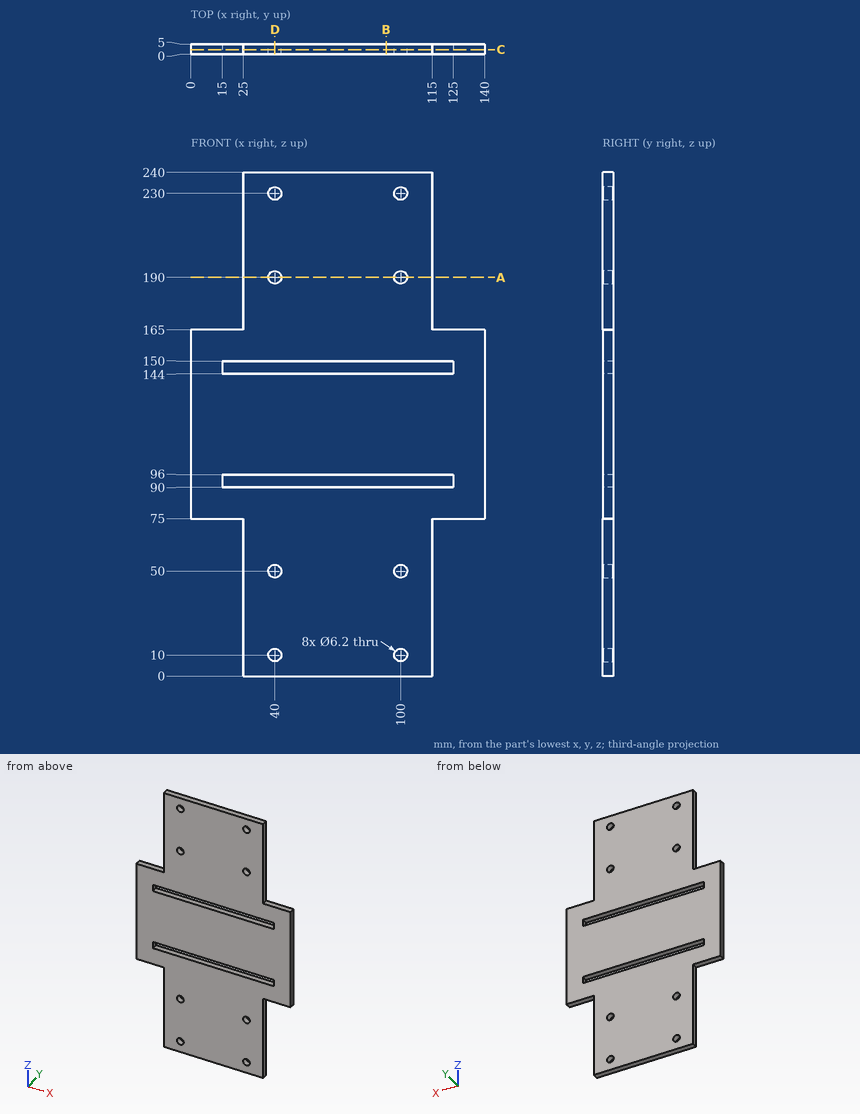
Verification items for this drawing (mm, ordinates from the low corner). Give positions to 0.01 mm unless a question says otherwise; leave off trailing zeros. Write each loop counter-clockwise with the first axis right and the second up, starting at its lowest first coordinate (ties: lowest second). Pieces come first, ordered by that corner, then holes.
1) Section check C-C, the plane y = 2.3. State how many separate pieces and enclosed holes the cut face has, and give its area (3 significant figures).
2) Section check D-D, the plane x = 40. Record the boundary of the cut face in (y, z).
3) Gauge pin test, flat end, axial feed: pin 1 (1.5 mm diameter, centred on y = 3.5, z = 215.5, fed in from +X). Record the tip position at first contact, or that the pin passes through.
4) Section check B-B, the plane x = 93. Record the boundary of the cut face in (y, z), and give its area (3 significant figures).
5) Section check A-A, the plane z = 190. Record the boundary of the cut face in (x, y), and give its area (3 significant figures).
6) Material ranges on L1, parallel to Z at x = 122, y = 1.65; L2, parallel to X at y = 1.7, z = 190; L3, parallel to Z at x = 28.5, y = 0.75, recorded low to high.
Computed:
1. separate pieces: 1
1. enclosed holes: 10
1. area: 24,500 mm2
2. outline: (0, 0) - (5, 0) - (5, 6.9) - (0, 6.9) - close; (0, 13.1) - (5, 13.1) - (5, 46.9) - (0, 46.9) - close; (0, 53.1) - (5, 53.1) - (5, 90) - (0, 90) - close; (0, 96) - (5, 96) - (5, 144) - (0, 144) - close; (0, 150) - (5, 150) - (5, 186.9) - (0, 186.9) - close; (0, 193.1) - (5, 193.1) - (5, 226.9) - (0, 226.9) - close; (0, 233.1) - (5, 233.1) - (5, 240) - (0, 240) - close
3. pin 1: stops at x = 115
4. outline: (0, 0) - (5, 0) - (5, 90) - (0, 90) - close; (0, 96) - (5, 96) - (5, 144) - (0, 144) - close; (0, 150) - (5, 150) - (5, 240) - (0, 240) - close
4. area: 1,140 mm2
5. outline: (25, 0) - (36.9, 0) - (36.9, 5) - (25, 5) - close; (43.1, 0) - (96.9, 0) - (96.9, 5) - (43.1, 5) - close; (103.1, 0) - (115, 0) - (115, 5) - (103.1, 5) - close
5. area: 388 mm2
6. L1: z = 75 to 90, 96 to 144, 150 to 165
6. L2: x = 25 to 36.9, 43.1 to 96.9, 103.1 to 115
6. L3: z = 0 to 90, 96 to 144, 150 to 240
